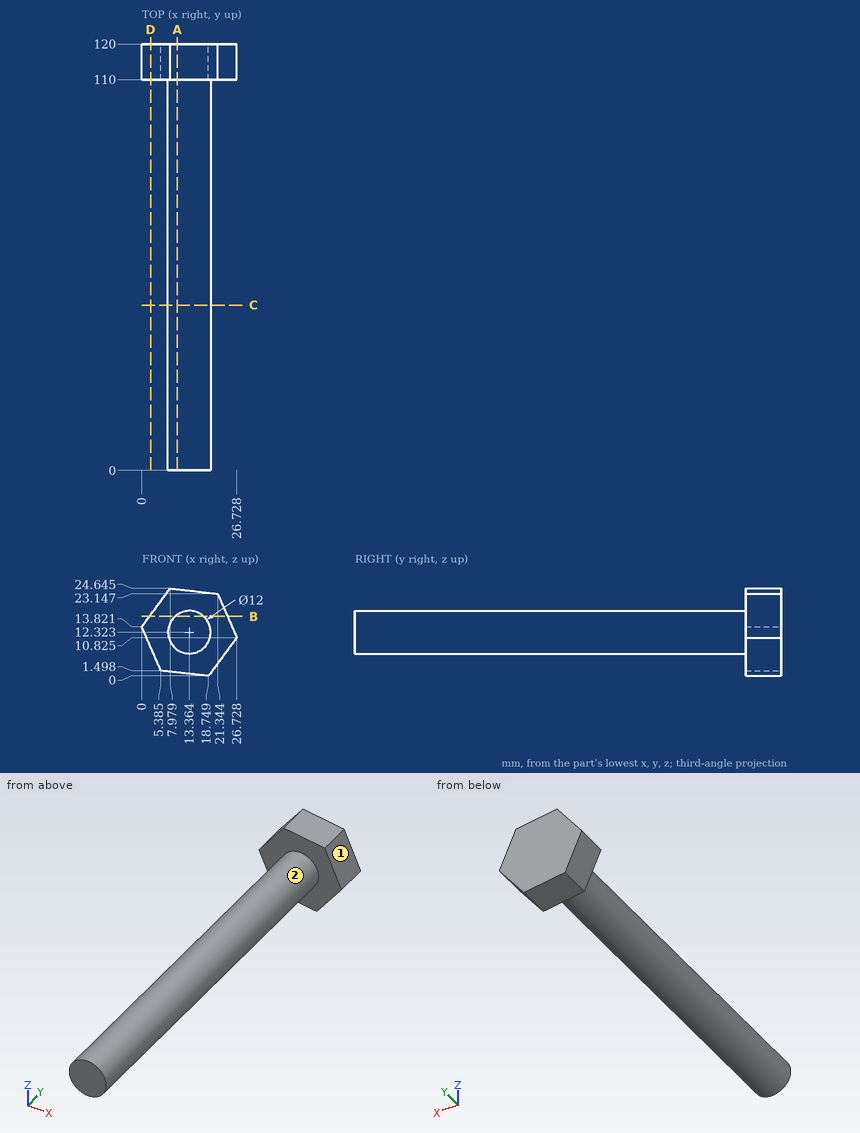
Answer from the drawing. Dimensions are ordinates in mm from the lowest x, y and z of the part. A direction names the side the tool comes from. Coordinates: 2 decimals unless noted, no trailing zeros. Write each loop counter-clockwise with the first axis right and the second up, starting at its lowest first coordinate (ties: lowest second). Pieces come first, ordered by that corner, then holes. Notation, with made-up numbers: (36, 10.25) - (68, 10.25) arc R21 cw to (68, 15.25) - close; hole circle Ø3 at (-29, -4). An arc over 180 degrees is marked (long way). Return JSON: item names as keys, results as strings.
1. The part is cut by section A-A on x = 10. Determine the outline of the cut face in (y, z) (1 decimal).
Final values:
{"outline": "(0, 7.4) - (110, 7.4) - (110, 1) - (120, 1) - (120, 24.4) - (110, 24.4) - (110, 17.3) - (0, 17.3) - close"}
2. Which of the six approach directions +Z, -Z, +X, -X, +Y, -Y give full straight-line access (tool end or side, diameter ignored) to the marked faces 1 and 2?
Final values:
{"face 1": "+Z, +X, +Y, -Y", "face 2": "-Y"}
3. The part is cut by section B-B on z = 16.75. Determine the outline of the cut face in (x, y) (1 decimal).
Final values:
{"outline": "(2.2, 110) - (9.3, 110) - (9.3, 0) - (17.4, 0) - (17.4, 110) - (24.1, 110) - (24.1, 120) - (2.2, 120) - close"}
4. Each of these flat-tipped pins is pushed along its axis until it touches: pin 1 Ø1 at (y, z) = (94, 9) entering from +X; pin 2 Ø7.5 at (x, z) = (19, 16) entering from -Y; pin 3 Ø3 at (y, z) = (12, 13) entering from +X; pin 4 Ø2 at (y, z) = (85, 8) entering from +X. Where does it stop, or does it pass through?
Final values:
{"pin 1": "x = 18.66", "pin 2": "y = 0", "pin 3": "x = 19.36", "pin 4": "x = 18.36"}
5. Consider line 1 along Y through (x, z) = (8.25, 21); line 2 along X through (y, z) = (105, 12.25) (1 decimal); line 3 along Z through (x, y) = (13.5, 113.5). Determine where each line is inside the solid, lowest interval first.
Final values:
{"line 1": "110 to 120", "line 2": "7.4 to 19.4", "line 3": "0.59 to 24.03"}
6. The part is cut by section D-D on x = 2.5. Determine the outline of the cut face in (y, z).
Final values:
{"outline": "(110, 8.1) - (120, 8.1) - (120, 17.21) - (110, 17.21) - close"}
7. The part is cut by section C-C on y = 46.5. Determine the outline of the cut face in (x, z) (1 decimal).
Final values:
{"outline": "circle Ø12 at (13.4, 12.3)"}
